Here's how the part is built. I have some questions about the finished solid (model axes, mm). A direction names the side the tool comes from. Coordinates: 2 decimals unless noted, no trailing zeros. Loops run counter-clockwise (first coordinate to the right, second up) from the corner with the lowest first, then second, coordinate; pieces in that order, holes last.
```python
from build123d import *

# Parameters (mm, degrees)
SKETCH1_W           = 431.8
SKETCH1_H           = 736.6
SKETCH1_W_2         = 401.32
SKETCH1_H_2         = 706.12
SKETCH1_H_3         = 15.24
BOSS_EXTRUDE1_DEPTH = 558.8
SKETCH3_W           = 584.2
SKETCH3_H           = 820.42
BOSS_EXTRUDE2_DEPTH = 20.32
SKETCH4_W           = 101.6
SKETCH4_H           = 25.4
CUT_EXTRUDE1_DEPTH  = 12.7
CUT_EXTRUDE2_DEPTH  = 7.62
FILLET1_R           = 7.46
FILLET2_R           = 2.54
SKETCH6_R           = 2.54
CUT_EXTRUDE3_DEPTH  = 9.906


with BuildPart() as part:
    # Sketch1 → Boss-Extrude1 (new body)
    # profile 1 of 2: a face of its own
    with BuildSketch(Plane.XY):
        Rectangle(SKETCH1_W, SKETCH1_H)
        Rectangle(SKETCH1_W_2, SKETCH1_H_2, mode=Mode.SUBTRACT)
    # profile 2 of 2: a face of its own
    with BuildSketch(Plane.XY):
        Rectangle(SKETCH1_W_2, SKETCH1_H_3)
    extrude(amount=BOSS_EXTRUDE1_DEPTH)

    # Sketch3 → Boss-Extrude2 (add)
    with BuildSketch(Plane(origin=(215.9, 0, 0), x_dir=(0, 0, -1), z_dir=(1, 0, 0))):
        with Locations((-279.4, -10.16)):
            Rectangle(SKETCH3_W, SKETCH3_H)
    extrude(amount=-BOSS_EXTRUDE2_DEPTH)

    # Sketch4 → Cut-Extrude1 (cut)
    with BuildSketch(Plane(origin=(215.9, 0, 0), x_dir=(0, 0, -1), z_dir=(1, 0, 0))):
        with Locations((-279.4, 347.087877014)):
            Rectangle(SKETCH4_W, SKETCH4_H)
    extrude(amount=-CUT_EXTRUDE1_DEPTH, mode=Mode.SUBTRACT)

    # Sketch5 → Cut-Extrude2 (cut)
    with BuildSketch(Plane.XZ.offset(-359.787877014)):
        Polygon((211.571045912, 228.6), (211.571045912, 330.2), (207.242091825, 330.2), (203.2, 330.2), (203.2, 228.6), (207.242091825, 228.6), align=None)
    extrude(amount=-CUT_EXTRUDE2_DEPTH, mode=Mode.SUBTRACT)

    # Fillet1
    # the kernel refuses this fillet: 7.46 mm, written as the material it takes off along each edge
    with BuildSketch(Plane(origin=(211.571045912, 359.787877014, 228.6), x_dir=(0, 1, 0), z_dir=(0, 0, 1))) as fillet1_piece_1:
        with BuildLine():
            CenterArc((6.771126309, -7.46), FILLET1_R, 90, 65.183641266)
            Line((0, -4.328954088), (-0.135422526, -4.266333169))
            ThreePointArc((-0.135422526, -4.266333169), (-0.1492, -2.164477044), (-0.1492, 0))
            Line((-0.1492, 0), (0, 0.1492))
            Line((0, 0.1492), (6.771126309, 0.1492))
            Line((6.771126309, 0.1492), (6.771126309, 0))
        make_face()
    extrude(amount=101.6, mode=Mode.SUBTRACT)

    # Fillet2
    fillet2_edges = [part.edges().sort_by_distance(p)[0] for p in [
        (211.571045912, 367.407877014, 279.4),
    ]]
    fillet(fillet2_edges, radius=FILLET2_R)

    # Sketch6 → Cut-Extrude3 (cut)
    with BuildSketch(Plane.ZY.offset(215.9)):
        with Locations((441.685832518, 330.962)):
            Circle(SKETCH6_R)
        with Locations((401.553832518, 330.962)):
            Circle(SKETCH6_R)
        with Locations((421.619832518, 315.976)):
            Circle(SKETCH6_R)
        with Locations(Location((137.180167482, 315.976, 0), (0, 0, 180))):
            Circle(SKETCH6_R)
        with Locations(Location((157.246167482, 330.962, 0), (0, 0, 180))):
            Circle(SKETCH6_R)
        with Locations(Location((117.114167482, 330.962, 0), (0, 0, 180))):
            Circle(SKETCH6_R)
    extrude(amount=-CUT_EXTRUDE3_DEPTH, mode=Mode.SUBTRACT)


solid = part.part
```
1. I want a section at C-C (z = 102). Please give me the cut outline in (x, y).
2. For pin 1 (1.5 mm diameter, centred on y = 315, z = 137.5, fed in from -X); pin 2 (3 mm diameter, centred on x = 101, z = 506.5, fed in from -Y), each with a flat end and sliding along its axis, tell me the tip position at first contact or that it passes through.
3. We'd pull the mould along Z, two halves only. Please class faces 4 (the flat face through (206, -16, -12.7)), 5 (the flat face through (203.2, 351, 280)), 6 (the flat face through (195.58, -96, 283)), 7 (the flat face through (-72, 2, 558.8)): +Z half, -Z half, draft (parallel to the pull), parting line (faces both ways), or undercut.
4. I want a section at B-B (x = -16). Please give me the cut outline in (y, z).
5. I need wall thicknesses on line 1 along Y through (x, z) = (9, 441.5); line 2 along X through (y, z) = (-214, 173.5). Which ranges of each line are inside material? Lowest first, please.
6. On a 3-axis mill with a long thin cutter (end or side, diameter ignored), from which of +Z, -Z, +X, -X, +Y, -Y can I reach the whole of each face in a straight line? I mean faces 1 (the flat face through (-72, 2, 0)), 2 (the flat face through (-5, -7.62, 275)), 3 (the flat face through (-13, 368.3, 275)). Say none if no direction works.
7. I want a section at A-A (y = 157.5). Please give me the cut outline in (x, z).
Response values:
1. outline: (-215.9, -368.3) - (195.58, -368.3) - (195.58, -420.37) - (215.9, -420.37) - (215.9, 400.05) - (195.58, 400.05) - (195.58, 368.3) - (-215.9, 368.3) - close; hole (-200.66, -353.06) - (195.58, -353.06) - (195.58, -7.62) - (-200.66, -7.62) - close; hole (-200.66, 7.62) - (195.58, 7.62) - (195.58, 353.06) - (-200.66, 353.06) - close
2. pin 1: stops at x = -205.99
2. pin 2: stops at y = -368.3
3. face 4: -Z half
3. face 5: undercut
3. face 6: draft
3. face 7: +Z half
4. outline: (-368.3, 0) - (-353.06, 0) - (-353.06, 558.8) - (-368.3, 558.8) - close; (-7.62, 0) - (7.62, 0) - (7.62, 558.8) - (-7.62, 558.8) - close; (353.06, 0) - (368.3, 0) - (368.3, 558.8) - (353.06, 558.8) - close
5. line 1: y = -368.3 to -353.06, -7.62 to 7.62, 353.06 to 368.3
5. line 2: x = -215.9 to -200.66, 195.58 to 215.9
6. face 1: -Z, -X, +Y, -Y
6. face 2: +Z, -Z
6. face 3: +Z, -Z, -X, +Y
7. outline: (-215.9, 0) - (-200.66, 0) - (-200.66, 558.8) - (-215.9, 558.8) - close; (195.58, -12.7) - (215.9, -12.7) - (215.9, 571.5) - (195.58, 571.5) - close
